```python
from build123d import *

# Parameters (mm, degrees)
F0_R     = 5
F1_DEPTH = 98
F2_W     = 4.8668145407
F2_H     = 4.5
F2_W_2   = 5.1924452364
F3_DEPTH = 12.5
F4_SIZE  = 1
F5_SIZE  = 1


with BuildPart() as f1:
    # F0 (on Top) → F1 (new body)
    with BuildSketch(Plane.XY):
        with Locations((-1.1064895812, 0)):
            Circle(F0_R)
    extrude(amount=F1_DEPTH)

    # F2 (on Right) → F3 (cut, symmetric)
    with BuildSketch(Plane.YZ):
        with Locations((5.3834072703, 95.75)):
            Rectangle(F2_W, F2_H)
        with Locations((-5.5462226182, 95.75)):
            Rectangle(F2_W_2, F2_H)
    extrude(amount=F3_DEPTH, both=True, mode=Mode.SUBTRACT)

    # F4
    f4_edges = [f1.edges().sort_by_distance(p)[0] for p in [
        (3.646672, -1.551599, 98),
        (-6.10649, 0, 98),
        (3.646672, 1.551599, 98),
    ]]
    chamfer(f4_edges, length=F4_SIZE)

    # F5
    f5_edges = [f1.edges().sort_by_distance(p)[0] for p in [
        (-6.10649, 0, 0),
    ]]
    chamfer(f5_edges, length=F5_SIZE)


solid = f1.part
```
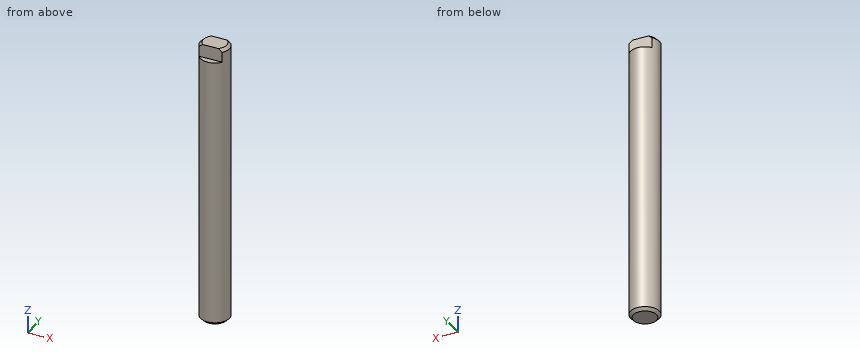
Check sheet for the modelled part. Datum: model origin and axes. Units: mm. Coordinates: 2 decimals unless noted, no trailing zeros. Loops run counter-clockwise (first coordinate to the right, second up) from the corner with the lowest first, then second, coordinate; pieces in that order, holes last. Notation, with made-up numbers: M 38.5,2 L 74.5,2 A34 cw 74.5,38 Z; hole C 46,70 d10. An arc over 180 degrees is marked long. Answer as a JSON object with one key per item and string values.
1. Sectioned sample at A-A on z = 52.5. Record the cut outline in (x, y).
Outcome:
{"outline": "C -1.11,0 d10"}
2. Depth check by flat-ended pin: P1, Ø5, axis at x = 2.5, z = 61.5, coming from the +Y side; P2, Ø2, axis at x = -2.5, z = 96.5, coming from the -Y side; P3, Ø1, axis at x = -1, y = 4.5, coming from the +Z side. Enter the tip coordinate at first touch or a pass-through.
Outcome:
{"P1": "y = 4.88", "P2": "y = -2.95", "P3": "z = 93.5"}
3. Scan lines: L1, parallel to Z at x = -3.25, y = -3.25; L2, parallel to X at y = -2.75, z = 52.5; L3, parallel to Y at x = -4, z = 63. Record each from-to range of solid material in increasing order. Write a range as from..to.
Outcome:
{"L1": "0..93.5", "L2": "-5.28..3.07", "L3": "-4.08..4.08"}
